```python
from build123d import *

# Parameters (mm, degrees)
PAD_DEPTH     = 15
FILLET_R      = 3
SKETCH001_R   = 6.125
HOLE_DEPTH    = 30.001
SKETCH002_R   = 2.625
HOLE001_DEPTH = 35.001


with BuildPart() as part:
    # Sketch → Pad (new body, symmetric)
    with BuildSketch(Plane.XY):
        with BuildLine():
            Line((-17.5, 0), (-17.5, -12.5))
            Line((-17.5, -12.5), (17.5, -12.5))
            Line((17.5, -12.5), (17.5, 0))
            ThreePointArc((17.5, 0), (0, 17.5), (-17.5, 0))
        make_face()
    extrude(amount=PAD_DEPTH, both=True)

    # Fillet
    fillet_edges = [part.edges().sort_by_distance(p)[0] for p in [
        (0, -12.5, 15),
    ]]
    fillet(fillet_edges, radius=FILLET_R)

    # Sketch001 (on Face5 of Fillet) → Hole (cut, through all)
    with BuildSketch(Plane.XY.offset(15)):
        with Locations((0, 2.5)):
            Circle(SKETCH001_R)
    extrude(amount=-HOLE_DEPTH, mode=Mode.SUBTRACT)

    # Sketch002 (on Face7 of Hole) → Hole001 (cut, through all)
    with BuildSketch(Plane.YZ.offset(17.5)):
        with Locations((2.5, 0)):
            Circle(SKETCH002_R)
    extrude(amount=-HOLE001_DEPTH, mode=Mode.SUBTRACT)


solid = part.part
```
Source: CAD feature listing. Evaluate the final solid. Frame: model axes, mm. Round coordinates to 2 decimals unless told otherwise and drop trailing zeros. Loops run counter-clockwise (first coordinate to the right, second up) from the corner with the lowest first, then second, coordinate; pieces in that order, holes last.
(1) Material intervals for probe 1 along Y at (x, z) = (0, -9) (3 decimals); probe 2 along Z at (x, y) = (-11.25, 2.5) (3 decimals); probe 3 along Y at (x, z) = (-3, 1), sorted ascending.
From the geometry:
probe 1: y = -12.5 to -3.625, 8.625 to 17.5
probe 2: z = -15 to -2.625, 2.625 to 15
probe 3: y = -12.5 to -2.84, 7.84 to 17.24
(2) Section query D-D (y = 4). Output: boundary loops of the cut face in (x, z), and give its area (3 significant figures).
From the geometry:
outline: (-17.04, -15) - (-5.94, -15) - (-5.94, -2.15) - (-17.04, -2.15) - close; (-17.04, 2.15) - (-5.94, 2.15) - (-5.94, 15) - (-17.04, 15) - close; (5.94, -15) - (17.04, -15) - (17.04, -2.15) - (5.94, -2.15) - close; (5.94, 2.15) - (17.04, 2.15) - (17.04, 15) - (5.94, 15) - close
area: 570 mm2
(3) Section query B-B (y = 8). Output: boundary loops of the cut face in (x, z), and give its area (3 significant figures).
From the geometry:
outline: (-15.56, -15) - (-2.7, -15) - (-2.7, 15) - (-15.56, 15) - close; (2.7, -15) - (15.56, -15) - (15.56, 15) - (2.7, 15) - close
area: 772 mm2
(4) Section query A-A (x = 0). Output: boundary loops of the cut face in (y, z) (3 decimals), and give its area (3 significant figures).
From the geometry:
outline: (-12.5, -15) - (-3.625, -15) - (-3.625, 15) - (-9.5, 15) arc R3 ccw to (-12.5, 12) - close; (8.625, -15) - (17.5, -15) - (17.5, 15) - (8.625, 15) - close
area: 531 mm2
(5) Contact query for flat-ended pins moving along their axis: pin 1 Ø6 at (y, z) = (7.5, -9) entering from +X; pin 2 Ø10 at (x, y) = (0, 2.5) entering from -Z; pin 3 Ø3 at (x, z) = (-7, -7.5) entering from +Y. Output: stop coordinate, or through.
From the geometry:
pin 1: stops at x = 16.91
pin 2: passes through
pin 3: stops at y = 16.61
(6) Pull-direction query (Z, two-part tool) for faces 1 (the cylindrical face through (-11.433, 1.931, -2.563)), 2 (the flat face through (0, -12.5, -1)), 3 (the flat face through (0, -5, 15)); classes: +Z half, -Z half, draft (parallel to the pull), parting line (faces both ways), or undercut.
From the geometry:
face 1: undercut
face 2: draft
face 3: +Z half
(7) Section query C-C (z = 0). Output: boundary loops of the cut face in (x, y) (3 decimals).
From the geometry:
outline: (-17.5, -12.5) - (17.5, -12.5) - (17.5, -0.125) - (5.534, -0.125) arc R6.125 cw to (-5.534, -0.125) - (-17.5, -0.125) - close; (-16.733, 5.125) - (-5.534, 5.125) arc R6.125 cw to (5.534, 5.125) - (16.733, 5.125) arc R17.5 ccw to start
